from build123d import *

# Parameters (mm, degrees)
F0_W      = 20.574
F0_H      = 20.574
F1_DEPTH  = 7.112
F2_W      = 17.018
F2_H      = 17.018
F3_DEPTH  = 5.334
F4_R      = 2.54
F5_W      = 5.588
F5_H      = 12.7
F6_DEPTH  = 3.048
F7_W      = 11.176
F7_H      = 12.7
F8_DEPTH  = 3.048
F9_R      = 2.6
F10_DEPTH = 1.778
F11_R     = 1.27
F12_R     = 1.27


with BuildPart() as f1:
    # F0 (on Top) → F1 (new body)
    with BuildSketch(Plane.XY):
        Rectangle(F0_W, F0_H)
    extrude(amount=F1_DEPTH)

    # F2 (on face) → F3 (cut)
    with BuildSketch(Plane(origin=(0, 0, 0), x_dir=(1, 0, 0), z_dir=(0, 0, -1))):
        Rectangle(F2_W, F2_H)
    extrude(amount=-F3_DEPTH, mode=Mode.SUBTRACT)

    # F4
    f4_edges = [f1.edges().sort_by_distance(p)[0] for p in [
        (-10.287, -10.287, 3.556),
        (10.287, 10.287, 3.556),
        (10.287, -10.287, 3.556),
        (-10.287, 10.287, 3.556),
    ]]
    fillet(f4_edges, radius=F4_R)

    # F5 (on face) → F6 (cut)
    with BuildSketch(Plane.XY.offset(7.112)):
        with Locations((-7.493, 0)):
            Rectangle(F5_W, F5_H)
    extrude(amount=-F6_DEPTH, mode=Mode.SUBTRACT)

    # F7 (on face) → F8 (cut)
    with BuildSketch(Plane.XY.offset(7.112)):
        with Locations((10.287, 0)):
            Rectangle(F7_W, F7_H)
    extrude(amount=-F8_DEPTH, mode=Mode.SUBTRACT)

    # F9 (on face) → F10 (cut)
    with BuildSketch(Plane.XY.offset(7.112)):
        Circle(F9_R)
    extrude(amount=-F10_DEPTH, mode=Mode.SUBTRACT)

    # F11
    f11_edges = [f1.edges().sort_by_distance(p)[0] for p in [
        (0, 10.287, 7.112),
        (0, -10.287, 7.112),
    ]]
    fillet(f11_edges, radius=F11_R)

    # F12
    f12_edges = [f1.edges().sort_by_distance(p)[0] for p in [
        (-10.287, 0, 0),
        (0, 10.287, 0),
        (-9.543051, 9.543051, 0),
    ]]
    fillet(f12_edges, radius=F12_R)


solid = f1.part
Model file for the job. Use its own axes, mm. A direction names the side the tool comes from. Coordinates: 2 decimals unless noted, no trailing zeros. Loops run counter-clockwise (first coordinate to the right, second up) from the corner with the lowest first, then second, coordinate; pieces in that order, holes last. Notation, with made-up numbers: (55.25, 59.25) -> (91.25, 59.25) arc R12 cw to (91.25, 80.25) -> close; hole circle Ø10 at (12, 52.25). An arc over 180 degrees is marked (long way). Use one line per item in the form item = value. Start each with the question number.
(1) Cut at D-D on z = 1.75. Give the cut face in (x, y), and give its area (3 significant figures).
(2) Tool access for faces 1 (the flat face through (4.699, 0, 6)), 2 (the flat face through (-4.699, 0, 6)), 3 (the flat face through (-8, 6.35, 6)), 4 (the flat face through (0, -8.509, 3)): list every direction of +Z, -Z, +X, -X, +Y, -Y with a clear straight run to the whole face (end or side of a thin tool).
(3) Cut at A-A on y = -3.75. Give the cut face in (x, z), and give its area (3 significant figures).
(4) Probe probe 1 along Y at (x, z) = (2.5, 4); probe 2 along Z at (x, y) = (-3.75, 4.75). List the from-to ranges inside material, lowest first. Write a range as from..to.
(5) Cut at C-C on y = 0. Give the cut face in (x, z), and give its area (3 significant figures).
(6) Pull direction X, two halves, no side cores. Call faces 5 (the cylindrical face through (9.905, 7.039, 6.75)), 6 (the cylindrical face through (-9.563, -9.523, 3.588)), 7 (the flat face through (-8.509, 0, 2)): pulls with the +X half, pulls with the -X half, needs draft (parallel to the pull), parting line crosses it, or undercut.
(7) Flat gauge pins, fed straight in: pin 1 (0.9 mm diameter, centred on x = -9.5, y = 0.5, fed in from +Z); pin 2 (3.5 mm diameter, centred on x = -8.5, z = 5, fed in from -Y); pin 3 (0.5 mm diameter, centred on y = 2, z = 6.5, fed in from -X); pin 4 (3 mm diameter, centred on x = 1.5, y = -5, fed in from -Z). Where does each tip first touch, or does it go through?
(8) Cut at B-B on x = 0. Give the cut face in (y, z).
Values:
q1.outline = (-10.29, -7.75) arc R2.54 ccw to (-7.75, -10.29) -> (7.75, -10.29) arc R2.54 ccw to (10.29, -7.75) -> (10.29, 7.75) arc R2.54 ccw to (7.75, 10.29) -> (-7.75, 10.29) arc R2.54 ccw to (-10.29, 7.75) -> close; hole (-8.51, -8.51) -> (8.51, -8.51) -> (8.51, 8.51) -> (-8.51, 8.51) -> close
q1.area = 128 mm2
q2.face_1 = +Z, -Z, +X
q2.face_2 = +Z, -Z, -X
q2.face_3 = +Z, -X
q2.face_4 = -Z
q3.outline = (-10.29, 1.27) arc R1.27 ccw to (-9.02, 0) -> (-8.51, 0) -> (-8.51, 4.06) -> (-10.29, 4.06) -> close; (-4.7, 5.33) -> (4.7, 5.33) -> (4.7, 7.11) -> (-4.7, 7.11) -> close; (8.51, 0) -> (9.02, 0) arc R1.27 ccw to (10.29, 1.27) -> (10.29, 4.06) -> (8.51, 4.06) -> close
q3.area = 30.5 mm2
q4.probe_1 = -10.29..-8.51, 8.51..10.29
q4.probe_2 = 5.33..7.11
q5.outline = (-10.29, 1.27) arc R1.27 ccw to (-9.02, 0) -> (-8.51, 0) -> (-8.51, 4.06) -> (-10.29, 4.06) -> close; (-4.7, 5.33) -> (-2.6, 5.33) -> (-2.6, 7.11) -> (-4.7, 7.11) -> close; (2.6, 5.33) -> (4.7, 5.33) -> (4.7, 7.11) -> (2.6, 7.11) -> close; (8.51, 0) -> (9.02, 0) arc R1.27 ccw to (10.29, 1.27) -> (10.29, 4.06) -> (8.51, 4.06) -> close
q5.area = 21.2 mm2
q6.face_5 = pulls with the +X half
q6.face_6 = pulls with the -X half
q6.face_7 = undercut
q7.pin_1 = 4.06
q7.pin_2 = -10.29
q7.pin_3 = -4.7
q7.pin_4 = 5.33
q8.outline = (-10.29, 1.27) arc R1.27 ccw to (-9.02, 0) -> (-8.51, 0) -> (-8.51, 5.33) -> (-2.6, 5.33) -> (-2.6, 7.11) -> (-9.02, 7.11) arc R1.27 ccw to (-10.29, 5.84) -> close; (2.6, 5.33) -> (8.51, 5.33) -> (8.51, 0) -> (9.02, 0) arc R1.27 ccw to (10.29, 1.27) -> (10.29, 5.84) arc R1.27 ccw to (9.02, 7.11) -> (2.6, 7.11) -> close
